```python
from build123d import *

# Parameters (mm, degrees)
F1_DEPTH = 92.964


with BuildPart() as f1:
    # F0 (on Top) → F1 (new body)
    with BuildSketch(Plane.XY):
        Polygon((-11.363891304, 28.6811531914), (-23.6685577262, 31.310043601), (-21.7514889919, 29.2647632039), (-21.4971445771, 29.1857769379), (-13.0953979351, 27.631865636), (-11.445167611, 28.3007349582), align=None)
        Polygon((-21.7514889919, 29.2647632039), (-23.6685577262, 31.310043601), (-35.158415116, 33.764850165), (-34.8719179356, 33.3392921913), align=None)
        Polygon((-21.7152671967, 29.2261189308), (-21.7514889919, 29.2647632039), (-34.8719179356, 33.3392921913), (-33.8031092464, 31.7517021871), (-31.0401167534, 30.9507590243), align=None)
        Polygon((-34.8719179356, 33.3392921913), (-35.158415116, 33.764850165), (-38.6320129037, 34.5069838887), align=None)
        Polygon((-10.8025132343, 28.5612148385), (-11.363891304, 28.6811531914), (-11.445167611, 28.3007349582), align=None)
        Polygon((-33.8031092464, 31.7517021871), (-34.8719179356, 33.3392921913), (-38.6320129037, 34.5069838887), (-56.4126817215, 38.3058215108), align=None)
        Polygon((-10.8025132343, 28.5612148385), (-11.445167611, 28.3007349582), (-11.6453689931, 27.3636813576), (-2.9640479419, 25.7580624939), (-2.536040841, 26.7950840673), align=None)
        Polygon((0, 32.9396761954), (-10.8025132343, 28.5612148385), (-2.536040841, 26.7950840673), align=None)
        Polygon((-18.2591771562, 25.5388890032), (-20.4559686533, 27.8825997451), (-31.0401167534, 30.9507590243), (-33.5801640761, 31.4205432739), (-29.339740332, 25.1218909351), (-26.0716256546, 22.3723570017), align=None)
        Polygon((-33.5801640761, 31.4205432739), (-31.0401167534, 30.9507590243), (-33.8031092464, 31.7517021871), align=None)
        Polygon((36.3568202391, 18.4856292647), (-2.536040841, 26.7950840673), (-2.9640479419, 25.7580624939), align=None)
        Polygon((-29.339740332, 25.1218909351), (-33.5801640761, 31.4205432739), (-37.7410697113, 32.190106862), align=None)
        Polygon((36.3568202391, 18.4856292647), (-2.9640479419, 25.7580624939), (-3.815611044, 23.6948039497), (26.957339273, 14.1383116556), (1.9335445611, 3.9956980087), (11.2069335345, -5.8978860567), (31.1385840178, 12.7843171358), align=None)
        Polygon((41.9932989192, 17.2813963145), (36.3568202391, 18.4856292647), (31.1385840178, 12.7843171358), (11.2069335345, -5.8978860567), (24.9195843935, -20.5276254565), align=None)
        Polygon((-27.1848988191, 21.921126494), (-29.339740332, 25.1218909351), (-37.7410697113, 32.190106862), (-50.2680484108, 34.5069838887), (-38.6320129037, 22.0927418237), (-39.6262408451, -9.3448986648), (-17.8473095251, -1.6648430482), (-16.271543508, 5.7106166242), align=None)
        Polygon((9.4679610689, -7.5278482606), (24.9195843935, -20.5276254565), (11.2069335345, -5.8978860567), align=None)
        Polygon((9.4679610689, -7.5278482606), (11.2069335345, -5.8978860567), (1.9335445611, 3.9956980087), (-2.2253809367, 2.3100074492), align=None)
        Polygon((0, -16.4022950937), (9.4679610689, -7.5278482606), (-2.2253809367, 2.3100074492), (-3.5101987058, 3.3909517865), (-13.6749758769, -0.1935240933), (-21.0544278002, -18.0732527887), align=None)
        Polygon((-21.0544278002, -18.0732527887), (-13.6749758769, -0.1935240933), (-17.8473095251, -1.6648430482), (-21.3581134797, -18.0973544137), align=None)
        Polygon((-21.3581134797, -18.0973544137), (-17.8473095251, -1.6648430482), (-39.6262408451, -9.3448986648), (-39.9497039616, -19.5728521794), align=None)
        Polygon((-21.6733533889, -19.5728521794), (-21.0544278002, -18.0732527887), (-21.3581134797, -18.0973544137), align=None)
    extrude(amount=F1_DEPTH)


solid = f1.part
```
Geometry: final body of the model. Coordinates: model frame, mm. A direction names the side the tool comes from. Round coordinates to 2 decimals unless told otherwise and drop trailing zeros. Write each loop counter-clockwise with the first axis right and the second up, starting at its lowest first coordinate (ties: lowest second). Pieces come first, ordered by that corner, then holes. Notation, with made-up numbers: M 51,-27.5 L 56,-27.5 A23 cw 56,-9.5 Z; hole C 0.5,-22 d4. An arc over 180 degrees is marked long. Answer in a Markdown table with one row per item. Add a question column.
(1) Cut plane B-B, the plane x = -15. Return the cut outline in (y, z).
(2) Reachability of faces 5 (the face through (4.668, -12.027, 45.831)), 6 (the face through (-45.266, 35.075, 45.831)), 7 (the face through (-5.33, 30.78, 45.83)) from +Z, -Z, +X, -X, +Y, -Y: full face, straight path, thin tool, end or side. Return the list, or none.
(3) Ray query, L1, parallel to Y at x = -3.5, z = 24; L2, parallel to X at y = -12, z = 81.5; L3, parallel to X at y = -9, z = 50. Return the intervals inside material, ascending.
(4) Cut plane A-A, the plane y = 10. Return the cut outline in (x, z), then the cut area to 3 significant figures.
(5) Draft query along X for faces 1 (the face through (-27.73, 23.77, 45.83)), 2 (the face through (-44.531, 28.387, 45.831)), 3 (the face through (3, 3, 0)), 4 (the face through (33.337, -1.888, 45.831)). Return one class per face: pulls with the +X half, pulls with the -X half, needs draft (parallel to the pull), parting line crosses it, or undercut.
(6) Contact query for flat-ended pins moving along their axis: pin 1 (3 mm diameter, centred on y = 21.5, z = 47, fed in from -X); pin 2 (1.5 mm diameter, centred on x = 12, z = 78, fed in from +Y); pin 3 (12 mm diameter, centred on x = -1, z = 60, fed in from -Y). Output: stop coordinate, or through.
(7) Cut plane C-C, the plane y = -6. Return the cut outline in (x, z).
Established:
| question | item | result |
|---|---|---|
| 1 | outline | M -17.59,0 L -0.66,0 L -0.66,92.96 L -17.59,92.96 Z; M 27.98,0 L 29.46,0 L 29.46,92.96 L 27.98,92.96 Z |
| 2 | face 5 | +Z, -Z, -Y |
| 2 | face 6 | +Z, -Z |
| 2 | face 7 | +Z, -Z, +Y |
| 3 | L1 | -16.68 to 3.38, 23.6 to 24.46, 25.86 to 31.52 |
| 3 | L2 | -39.71 to 4.7, 14.78 to 28.77 |
| 3 | L3 | -39.62 to 7.9, 11.22 to 30.13 |
| 4 | outline | M -39.01,0 L -19.16,0 L -19.16,92.96 L -39.01,92.96 Z; M 16.75,0 L 38.71,0 L 38.71,92.96 L 16.75,92.96 Z |
| 4 | area | 3,890 mm² |
| 5 | face 1 | undercut |
| 5 | face 2 | pulls with the -X half |
| 5 | face 3 | needs draft |
| 5 | face 4 | pulls with the +X half |
| 6 | pin 1 | x = -39.48 |
| 6 | pin 2 | y = 23.85 |
| 6 | pin 3 | y = -16.96 |
| 7 | outline | M -39.52,0 L 31.48,0 L 31.48,92.96 L -39.52,92.96 Z |
